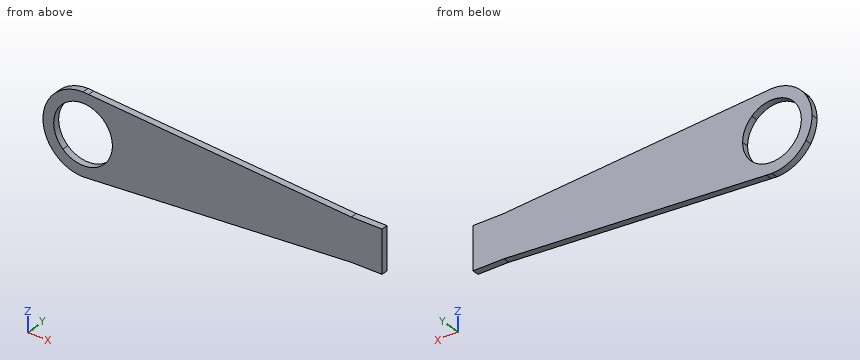
from build123d import *

# Parameters (mm, degrees)
SKETCH1_W           = 1.152195829
SKETCH1_H           = 1.6
BOSS_EXTRUDE3_DEPTH = 0.25


with BuildPart() as part:
    # Sketch1 → Boss-Extrude3 (new body)
    with BuildSketch(Plane(origin=(0, 0, 0), x_dir=(1, 0, 0), z_dir=(0, 1, 0))):
        with BuildLine():
            Line((-2.942295951, 1.981055848), (-3.150287356, 1.995545977))
            ThreePointArc((-3.150287356, 1.995545977), (-3.874856194, 1.808938531), (-4.41914511, 1.295545977))
            Line((-4.41914511, 1.295545977), (-3.9052708, 1.295545977))
            ThreePointArc((-3.9052708, 1.295545977), (-3.150287356, 1.595545977), (-2.395303913, 1.295545977))
            Line((-2.395303913, 1.295545977), (-1.881429602, 1.295545977))
            ThreePointArc((-1.881429602, 1.295545977), (-2.336191658, 1.755406364), (-2.942295951, 1.981055848))
        make_face()
        with BuildLine():
            Line((6.897516815, 1.295545977), (-2.942295951, 1.981055848))
            ThreePointArc((-2.942295951, 1.981055848), (-2.336191658, 1.755406364), (-1.881429602, 1.295545977))
            Line((-1.881429602, 1.295545977), (6.897516815, 1.295545977))
        make_face()
        with BuildLine():
            Line((-3.9052708, 1.295545977), (-4.41914511, 1.295545977))
            ThreePointArc((-4.41914511, 1.295545977), (-4.591343676, 0.91190722), (-4.650287356, 0.495545977))
            ThreePointArc((-4.650287356, 0.495545977), (-4.591343676, 0.079184734), (-4.41914511, -0.304454023))
            Line((-4.41914511, -0.304454023), (-3.9052708, -0.304454023))
            ThreePointArc((-3.9052708, -0.304454023), (-4.250287356, 0.495545977), (-3.9052708, 1.295545977))
        make_face()
        with BuildLine():
            ThreePointArc((-1.650287356, 0.495545977), (-1.709231037, 0.91190722), (-1.881429602, 1.295545977))
            Line((-1.881429602, 1.295545977), (-2.395303913, 1.295545977))
            ThreePointArc((-2.395303913, 1.295545977), (-2.140217609, 0.931159459), (-2.050287356, 0.495545977))
            ThreePointArc((-2.050287356, 0.495545977), (-2.140217609, 0.059932495), (-2.395303913, -0.304454023))
            Line((-2.395303913, -0.304454023), (-1.881429602, -0.304454023))
            ThreePointArc((-1.881429602, -0.304454023), (-1.709231037, 0.079184734), (-1.650287356, 0.495545977))
        make_face()
        with BuildLine():
            ThreePointArc((-2.395303913, -0.304454023), (-3.150287356, -0.604454023), (-3.9052708, -0.304454023))
            Line((-3.9052708, -0.304454023), (-4.41914511, -0.304454023))
            ThreePointArc((-4.41914511, -0.304454023), (-3.874856194, -0.817846577), (-3.150287356, -1.004454023))
            Line((-3.150287356, -1.004454023), (-2.942295951, -0.989963893))
            ThreePointArc((-2.942295951, -0.989963893), (-2.336191658, -0.76431441), (-1.881429602, -0.304454023))
            Line((-1.881429602, -0.304454023), (-2.395303913, -0.304454023))
        make_face()
        with BuildLine():
            Line((6.897516815, -0.304454023), (6.897516815, 1.295545977))
            Line((6.897516815, 1.295545977), (-1.881429602, 1.295545977))
            ThreePointArc((-1.881429602, 1.295545977), (-1.709231037, 0.91190722), (-1.650287356, 0.495545977))
            ThreePointArc((-1.650287356, 0.495545977), (-1.709231037, 0.079184734), (-1.881429602, -0.304454023))
            Line((-1.881429602, -0.304454023), (6.897516815, -0.304454023))
        make_face()
        with BuildLine():
            Line((-2.942295951, -0.989963893), (6.897516815, -0.304454023))
            Line((6.897516815, -0.304454023), (-1.881429602, -0.304454023))
            ThreePointArc((-1.881429602, -0.304454023), (-2.336191658, -0.76431441), (-2.942295951, -0.989963893))
        make_face()
        with Locations((7.47361473, 0.495545977)):
            Rectangle(SKETCH1_W, SKETCH1_H)
    extrude(amount=BOSS_EXTRUDE3_DEPTH)


solid = part.part
For this review, take the finished solid that the model builds, in its own axes (mm). Give positions to 0.01 mm unless a question says otherwise; leave off trailing zeros. Order: outer loops, then holes, each group sorted by start corner. A loop starts at its lowest first (then second) coordinate and runs counter-clockwise, first axis right, second up. Notation, with made-up numbers: M 9,65.25 L 50,65.25 A22 ccw 50,84.25 Z; hole C 31.5,-19.75 d9. An arc over 180 degrees is marked long. Answer in a Markdown table with one row per item. Add a question column.
(1) Consider section C-C on z = -0.6. State the section outline as (x, y) points.
(2) Wall thickness on probe 1 along X at (y, z) = (0.2, -1); probe 2 along Z at (x, y) = (-2.25, 0.2); probe 3 along X at (y, z) = (0.2, -0.3): over which ranges is each line inside the solid? List them lowest first. Write a range as [from, to].
(3) Consider section D-D on x = 6.25. State the section outline as (y, z) points, and give its area (3 significant figures).
(4) Consider section A-A on y = 0.05. State the section outline as (x, z) points, and give its area (3 significant figures).
(5) Consider section B-B on x = -2.5. State the section outline as (y, z) points.
Evaluation:
| question | item | result |
|---|---|---|
| 1 | outline | M -4.65,0 L -4.25,0 L -4.25,0.25 L -4.65,0.25 Z; M -2.06,0 L 8.05,0 L 8.05,0.25 L -2.06,0.25 Z |
| 2 | probe 1 | x = [-4.56, -4.13], [-2.17, 8.05] |
| 2 | probe 2 | z = [-1.93, -1.13], [0.14, 0.94] |
| 2 | probe 3 | x = [-4.64, -4.23], [-2.07, 8.05] |
| 3 | outline | M 0,-1.34 L 0.25,-1.34 L 0.25,0.35 L 0,0.35 Z |
| 3 | area | 0.423 mm^2 |
| 4 | outline | M -3.15,-2 L 6.9,-1.3 L 8.05,-1.3 L 8.05,0.3 L 6.9,0.3 L -3.15,1 A1.5 ccw Z; hole C -3.15,-0.5 d2.2 |
| 4 | area | 24.7 mm^2 |
| 5 | outline | M 0,-1.95 L 0.25,-1.95 L 0.25,-1.38 L 0,-1.38 Z; M 0,0.39 L 0.25,0.39 L 0.25,0.96 L 0,0.96 Z |
